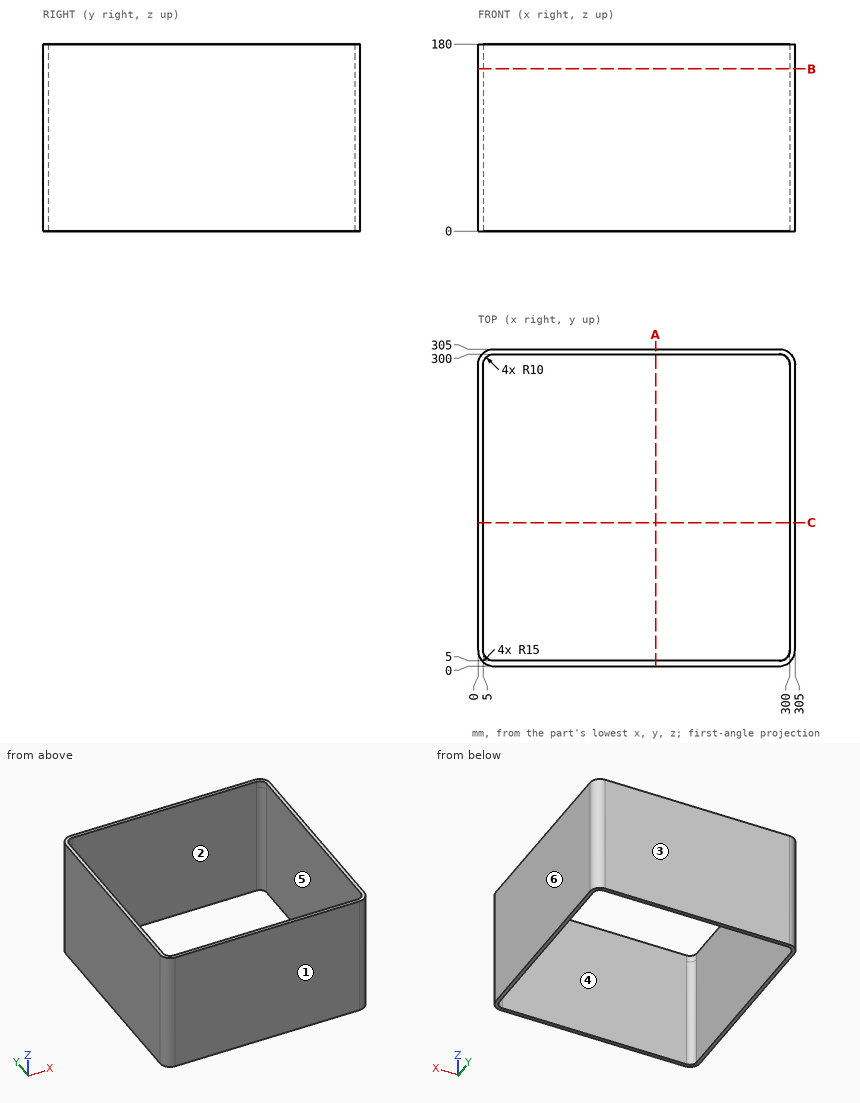
Check sheet for the drawn part. Datum: minimum x, y, z corner. Units: mm. A direction names the side the tool comes from. Give positions to 0.01 mm unless a question says otherwise; leave off trailing zeros. Order: outer loops, then holes, each group sorted by start corner. A loop starts at its lowest first (then second) coordinate and runs counter-clockwise, first axis right, second up. Notation, with made-up numbers: (39, -16) - (92, -16) arc R11 cw to (92, -9) - close; hole circle Ø6 at (-34.5, 58). An arc over 180 degrees is marked (long way). Write item = value, one per line. Start each with the question number.
1) Scan line: L1, parallel to X at y = 59, z = 134.5. Record every from-to range of solid material in increasing order.
2) Access from +Z, -Z, +X, -X, +Y, -Y to the whole of each face (thin tool, end or side, straight path). Record for the marked faces 5 and 6.
3) Section check B-B (z = 156). Enter the section's corners in (x, y).
4) Section check A-A (x = 171). Enter the section's corners in (y, z).
5) Gauge pin test, flat end, axial feed: pin 1 Ø5 at (x, z) = (38.5, 30) entering from -Y. Record the tip position at first contact, or that the pin passes through.
6) Draft check along Y on the marked faces 1, 2, 3 and 4. Enter one of: released by +Y, released by -Y, zero draft, split by the parting line, or undercut.
Geometry check:
q1.L1 = 0 to 5, 300 to 305
q2.face_5 = +Z, -Z
q2.face_6 = +Z, -Z, +X, +Y, -Y
q3.outline = (0, 15) arc R15 ccw to (15, 0) - (290, 0) arc R15 ccw to (305, 15) - (305, 290) arc R15 ccw to (290, 305) - (15, 305) arc R15 ccw to (0, 290) - close; hole (5, 15) arc R10 ccw to (15, 5) - (290, 5) arc R10 ccw to (300, 15) - (300, 290) arc R10 ccw to (290, 300) - (15, 300) arc R10 ccw to (5, 290) - close
q4.outline = (0, 0) - (5, 0) - (5, 180) - (0, 180) - close; (300, 0) - (305, 0) - (305, 180) - (300, 180) - close
q5.pin_1 = 0
q6.face_1 = released by -Y
q6.face_2 = undercut
q6.face_3 = released by +Y
q6.face_4 = undercut
